```python
from build123d import *

# Parameters (mm, degrees)
SKETCH_1_W               = 30
SKETCH_1_H               = 13
CUT_EXTRUDE_1_DEPTH      = 8
SKETCH_3_R               = 2.25
CUT_EXTRUDE_2_DEPTH      = 79.192071209
PATTERN_CIRCULAR_1_COUNT = 12
CHAMFER_1_SIZE           = 1
CHAMFER_2_SIZE           = 0.5
HOLE_WIZARD_M8_2_D       = 6.8
PATTERN_CIRCULAR_2_COUNT = 8
CUT_EXTRUDE_3_DEPTH      = 5
FILLET_1_R               = 1
HOLE_WIZARD_M3_1_D       = 2.5
HOLE_WIZARD_M3_1_DEPTH   = 7.5
HOLE_WIZARD_M3_1_TIP     = 0.751075774


with BuildPart() as part:
    # 草图1 → 旋转1 (revolve)
    with BuildSketch(Plane.XY, mode=Mode.PRIVATE) as revolve_1_sk:
        with Locations((-40, -6.5)):
            Rectangle(SKETCH_1_W, SKETCH_1_H)
    revolve(revolve_1_sk.sketch.rotate(Axis((0, 0, 0), (0, -1, 0)), 270), axis=Axis((0, 0, 0), (0, -1, 0)))

    # 草图2 → 切除-拉伸1 (cut)
    with BuildSketch(Plane(origin=(0, 0, 0), x_dir=(1, 0, 0), z_dir=(0, 1, 0))):
        with BuildLine():
            Line((4, 65.625784045), (4, 51))
            ThreePointArc((4, 51), (0, 47), (-4, 51))
            Line((-4, 51), (-4, 65.625784045))
            ThreePointArc((-4, 65.625784045), (0, 69.625784045), (4, 65.625784045))
        make_face()
    cut_extrude_1 = extrude(amount=-CUT_EXTRUDE_1_DEPTH, mode=Mode.SUBTRACT)

    # 草图3 → 切除-拉伸2 (cut, through all)
    with BuildSketch(Plane(origin=(0, -8, 0), x_dir=(1, 0, 0), z_dir=(0, 1, 0))):
        with Locations(Location((0, 51, 0), (0, 0, 270))):
            Circle(SKETCH_3_R)
    cut_extrude_2 = extrude(amount=-CUT_EXTRUDE_2_DEPTH, mode=Mode.SUBTRACT)

    # 阵列(圆周)1: 切除-拉伸1, 切除-拉伸2 ×12 about axis
    pattern_circular_1_axis = Axis((0, 0, 0), (0, 1, 0))
    add([cut_extrude_1.rotate(pattern_circular_1_axis, i * 360 / PATTERN_CIRCULAR_1_COUNT) for i in range(1, PATTERN_CIRCULAR_1_COUNT)], mode=Mode.SUBTRACT)
    add([cut_extrude_2.rotate(pattern_circular_1_axis, i * 360 / PATTERN_CIRCULAR_1_COUNT) for i in range(1, PATTERN_CIRCULAR_1_COUNT)], mode=Mode.SUBTRACT)

    # 倒角1
    chamfer_1_edges = [part.edges().sort_by_distance(p)[0] for p in [
        (0, 0, -25),
        (0, -13, -25),
    ]]
    chamfer(chamfer_1_edges, length=CHAMFER_1_SIZE)

    # 倒角2
    chamfer_2_edges = [part.edges().sort_by_distance(p)[0] for p in [
        (0, -13, -55),
    ]]
    chamfer(chamfer_2_edges, length=CHAMFER_2_SIZE)

    # M8 螺纹孔2 (through all)
    with Locations(Plane(origin=(0, 0, 0), x_dir=(1, 0, 0), z_dir=(0, 1, 0))):
        with Locations((35.25629266, 9.446895146)):
            hole_wizard_m8_2 = Hole(HOLE_WIZARD_M8_2_D / 2)

    # 阵列(圆周)2: M8 螺纹孔2 ×8 about axis
    pattern_circular_2_axis = Axis((0, 0, 0), (0, 1, 0))
    for i in range(1, PATTERN_CIRCULAR_2_COUNT):
        add(hole_wizard_m8_2.rotate(pattern_circular_2_axis, i * 360 / PATTERN_CIRCULAR_2_COUNT), mode=Mode.SUBTRACT)

    # 草图8 → 切除-拉伸3 (cut)
    with BuildSketch(Plane.XZ.offset(13)):
        Polygon((-21.727676324, -22.402412405), (-14.422539176, -12.882172321), (-8.710395126, -17.26525461), (-16.015532274, -26.785494693), align=None)
    extrude(amount=-CUT_EXTRUDE_3_DEPTH, mode=Mode.SUBTRACT)

    # 圆角1
    fillet_1_edges = [part.edges().sort_by_distance(p)[0] for p in [
        (-16.015532274, -10.5, -26.785494693),
        (-21.727676324, -10.5, -22.402412405),
    ]]
    fillet(fillet_1_edges, radius=FILLET_1_R)

    # M3 螺纹孔1
    with Locations(Plane(origin=(0, -8, 0), x_dir=(-1, 0, 0), z_dir=(0, -1, 0))):
        with Locations((16.436558583, 21.420540188)):
            Hole(HOLE_WIZARD_M3_1_D / 2, depth=HOLE_WIZARD_M3_1_DEPTH)
            with Locations((0, 0, -(HOLE_WIZARD_M3_1_DEPTH + HOLE_WIZARD_M3_1_TIP / 2))):  # 118° drill point
                Cone(0, HOLE_WIZARD_M3_1_D / 2, HOLE_WIZARD_M3_1_TIP, mode=Mode.SUBTRACT)


solid = part.part
```
CAD build for the part. Positions are in the model's coordinates, mm. A direction names the side the tool comes from. Coordinates: 2 decimals unless noted, no trailing zeros. Order: outer loops, then holes, each group sorted by start corner. A loop starts at its lowest first (then second) coordinate and runs counter-clockwise, first axis right, second up.
(1) Saw through at A-A, the plane x = 0. Write the cut outline in (y, z), and give its area (3 significant figures).
Solution:
outline: (-13, -54.5) - (-12.5, -55) - (-8, -55) - (-8, -53.25) - (-13, -53.25) - close; (-13, -48.75) - (-8, -48.75) - (-8, -47) - (0, -47) - (0, -26) - (-1, -25) - (-12, -25) - (-13, -26) - close; (-13, 26) - (-12, 25) - (-1, 25) - (0, 26) - (0, 47) - (-8, 47) - (-8, 48.75) - (-13, 48.75) - close; (-13, 53.25) - (-8, 53.25) - (-8, 55) - (-12.5, 55) - (-13, 54.5) - close
area: 605 mm2
(2) Which spindle directions (+Z, -Z, +X, -X, +Y, -Y) get a long thin tool onto all of the face, cutting with end or side? Do faces 1 (the face through (45, -8, -28)), 2 (the face through (23.013, -3.944, 47.86)), 3 (the face through (-13.8, -10.5, -23.9)), 4 (the face through (0, -4, -47)). Say none if no direction does.
Solution:
face 1: +Y
face 2: +X, +Y
face 3: -Y
face 4: -Z, +Y
(3) Mould opens along X. For faces 5 (the face through (43.86, -3.94, 29.94)), 6 (the face through (-23.58, -3.94, 40.66)), 7 (the face through (-53, -4, -4)), 8 (the face through (-47, -4, 0)) say: released by +X, released by -X, zero draft, split by the parting line, or undercut.
Solution:
face 5: released by +X
face 6: undercut
face 7: zero draft
face 8: released by -X
(4) Pin check, flat tips, straight feed: pin 1 Ø4 at (x, z) = (-1, -53) entering from +Y; pin 2 Ø1 at (y, z) = (-2, 22.5) entering from +X; pin 3 Ø1.5 at (x, y) = (30, -2) entering from +Z. Stop position of each tip, or through.
Solution:
pin 1: stops at y = -8
pin 2: stops at x = 50.41
pin 3: stops at z = 45.26
(5) Saw through at B-B, the plane z = 18.25. Count the separate pieces of the cut face and the enclosed holes in it, and give its area (3 significant figures).
Solution:
separate pieces: 3
enclosed holes: 0
area: 813 mm2
(6) Drill centre lines: L1, parallel to Z at x = -25.5, y = -10.6; L2, parallel to Z at x = 11.5, y = -9. Where is each one in solid material? Low to high.
Solution:
L1: z = -48.73 to -46.42, -41.92 to 41.92, 46.42 to 48.73
L2: z = -53.78 to -22.2, 22.2 to 32.55, 37.97 to 53.78
